Answer from the drawing. Dimensions are ordinates in mm from the lowest x, y and z of the part. A direction names the side the tool comes from. Give positions to 0.01 mm unless a question says otherwise; leave off trailing zeros. Order: outer loops, then holes, each group sorted by start corner. A loop starts at its lowest first (then second) coordinate and runs counter-clockwise, first axis right, second up. Notation, with made-up numbers: (74, 42) - (100, 42) arc R18 ccw to (100, 77) - close; hole circle Ø2 at (73.25, 6.5). An arc over 180 degrees is marked (long way). Answer in a Markdown table with one row per item. Add a question column.
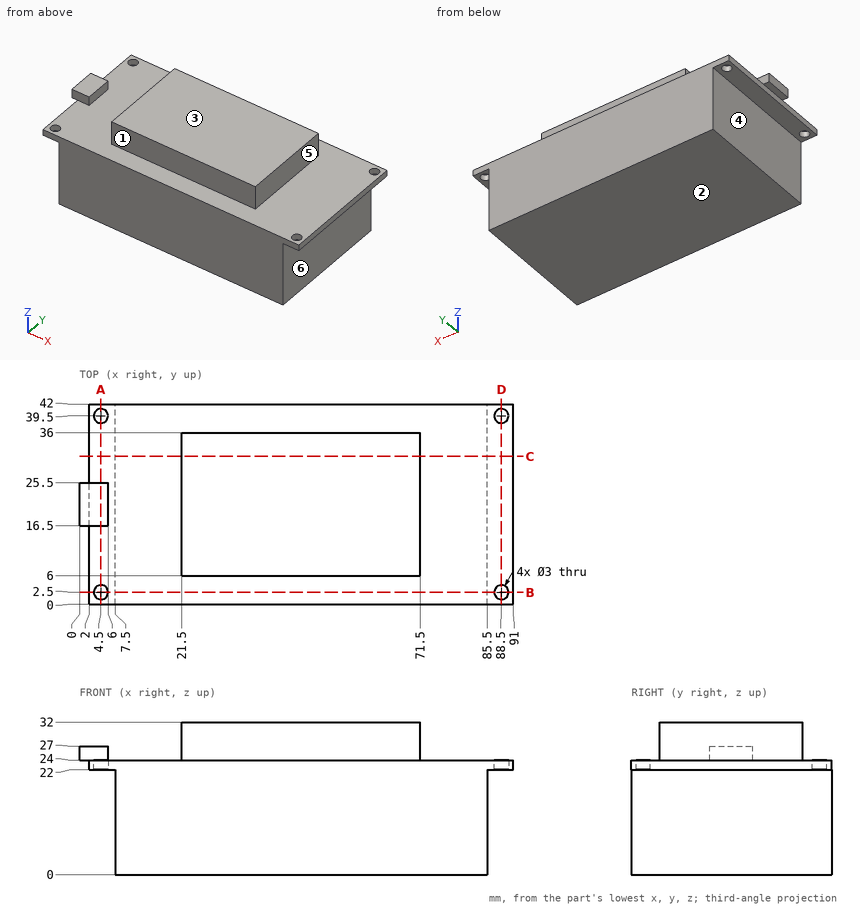
(1) Find section C-C, the plane y = 31. Write down the section's boundary in (x, z), plus the area to 3 significant figures.
(2) The mould has two halves that part along Z. Classify the marked faces 1, 2 and 3: +Z half, -Z half, draft (parallel to the pull), parting line (faces both ways), or undercut.
(3) Straight lines are drawn through the part: line 1 (Y direction, x = 4.5, z = 23.25); line 2 (Y direction, x = 4, z = 23); line 3 (Z direction, x = 82.5, y = 37.5). For each, find the intervals that lie inside material, in ascending order.
(4) Find section A-A, the plane x = 4.5. Write down the section's boundary in (y, z).
(5) Each of these flat-tipped pins is pushed along its axis until it touches: P1, Ø6.5, axis at y = 28, z = 12.5, coming from the -X side; P2, Ø3, axis at y = 33, z = 7, coming from the +X side; P3, Ø2.5, axis at x = 39, z = 27, coming from the +Y side. Where does it stop, or does it pass through?
(6) Find section B-B, the plane y = 2.5. Write down the section's boundary in (x, z), plus the area to 3 significant figures.
(7) For the marked faces 4, 5 and 6, determine the directions among +Z, -Z, +X, -X, +Y, -Y from which every point of the face is accessible in a straight line to the end or side of a thin tool.
(8) Find section D-D, the plane x = 88.5. Write down the section's boundary in (y, z), plus the area to 3 significant figures.
Answer key:
| question | item | result |
|---|---|---|
| 1 | outline | (2, 22) - (7.5, 22) - (7.5, 0) - (85.5, 0) - (85.5, 22) - (91, 22) - (91, 24) - (71.5, 24) - (71.5, 32) - (21.5, 32) - (21.5, 24) - (2, 24) - close |
| 1 | area | 2,290 mm² |
| 2 | face 1 | draft |
| 2 | face 2 | -Z half |
| 2 | face 3 | +Z half |
| 3 | line 1 | 0 to 1, 4 to 38, 41 to 42 |
| 3 | line 2 | 0 to 1.09, 3.91 to 38.09, 40.91 to 42 |
| 3 | line 3 | 0 to 24 |
| 4 | outline | (0, 22) - (1, 22) - (1, 24) - (0, 24) - close; (4, 22) - (38, 22) - (38, 24) - (25.5, 24) - (25.5, 27) - (16.5, 27) - (16.5, 24) - (4, 24) - close; (41, 22) - (42, 22) - (42, 24) - (41, 24) - close |
| 5 | P1 | x = 7.5 |
| 5 | P2 | x = 85.5 |
| 5 | P3 | y = 36 |
| 6 | outline | (2, 22) - (3, 22) - (3, 24) - (2, 24) - close; (6, 22) - (7.5, 22) - (7.5, 0) - (85.5, 0) - (85.5, 22) - (87, 22) - (87, 24) - (6, 24) - close; (90, 22) - (91, 22) - (91, 24) - (90, 24) - close |
| 6 | area | 1,880 mm² |
| 7 | face 4 | -Z, -X, +Y, -Y |
| 7 | face 5 | +Z, +X, +Y, -Y |
| 7 | face 6 | -Z, +X, +Y, -Y |
| 8 | outline | (0, 22) - (1, 22) - (1, 24) - (0, 24) - close; (4, 22) - (38, 22) - (38, 24) - (4, 24) - close; (41, 22) - (42, 22) - (42, 24) - (41, 24) - close |
| 8 | area | 72.0 mm² |
